```python
from build123d import *

# Parameters (mm, degrees)
SKETCH1_W           = 54
SKETCH1_H           = 13
SKETCH1_W_2         = 4
SKETCH1_H_2         = 4
BOSS_EXTRUDE1_DEPTH = 4


with BuildPart() as part:
    # Sketch1 → Boss-Extrude1 (new body)
    with BuildSketch(Plane.XY):
        with Locations((27, 6.5)):
            Rectangle(SKETCH1_W, SKETCH1_H)
        Polygon((7, 3), (7, 6), (47, 6), (47, 3), (45, 3), (45, 5), (37.5, 5), (37.5, 3), (35.5, 3), (35.5, 5), (28, 5), (28, 3), (26, 3), (26, 5), (18.5, 5), (18.5, 3), (16.5, 3), (16.5, 5), (9, 5), (9, 3), align=None, mode=Mode.SUBTRACT)
        with Locations((50.5, 6.5)):
            Rectangle(SKETCH1_W_2, SKETCH1_H_2, mode=Mode.SUBTRACT)
        with Locations((3.5, 6.5)):
            Rectangle(SKETCH1_W_2, SKETCH1_H_2, mode=Mode.SUBTRACT)
    extrude(amount=BOSS_EXTRUDE1_DEPTH)


solid = part.part
```
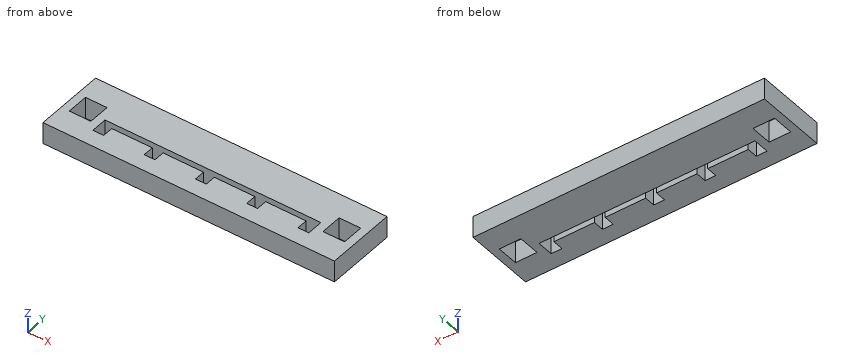
Model file for the job. Use its own axes, mm. Coordinates: 2 decimals unless noted, no trailing zeros. Order: outer loops, then holes, each group sorted by start corner. A loop starts at its lowest first (then second) coordinate and runs counter-clockwise, first axis right, second up. Notation, with made-up numbers: (47, 72) -> (72, 72) arc R26 cw to (72, 99) -> close; hole circle Ø11 at (7.5, 48). An arc over 180 degrees is marked (long way). Answer as a JSON object with one key per item and string values. Group by question number.
1) Cut at B-B, the plane y = 7.25. Write the cut outline in (x, z).
2) Drill centre lines: L1, parallel to X at y = 7.5, z = 3.85; L2, parallel to X at y = 3.5, z = 3.25; L3, parallel to Y at x = 21.5, z = 1.5. Where is each one in solid material? Low to high.
3) Cut at C-C, the plane z = 1.55. Count the separate pieces of the cut face and the enclosed holes in it, then the cut area to 3 significant figures.
4) Cut at A-A, the plane x = 5. Write the cut outline in (y, z).
5) Cut at D-D, the plane x = 34. Write the cut outline in (y, z).
Check values:
{
 "1": {"outline": "(0, 0) -> (1.5, 0) -> (1.5, 4) -> (0, 4) -> close; (5.5, 0) -> (48.5, 0) -> (48.5, 4) -> (5.5, 4) -> close; (52.5, 0) -> (54, 0) -> (54, 4) -> (52.5, 4) -> close"},
 "2": {"L1": "x = 0 to 1.5, 5.5 to 48.5, 52.5 to 54", "L2": "x = 0 to 7, 9 to 16.5, 18.5 to 26, 28 to 35.5, 37.5 to 45, 47 to 54", "L3": "y = 0 to 5, 6 to 13"},
 "3": {"separate pieces": "1", "enclosed holes": "3", "area": "610 mm²"},
 "4": {"outline": "(0, 0) -> (4.5, 0) -> (4.5, 4) -> (0, 4) -> close; (8.5, 0) -> (13, 0) -> (13, 4) -> (8.5, 4) -> close"},
 "5": {"outline": "(0, 0) -> (5, 0) -> (5, 4) -> (0, 4) -> close; (6, 0) -> (13, 0) -> (13, 4) -> (6, 4) -> close"}
}
